Read the model definition and answer for the solid it produces. Units are mm, in the model's axes. A direction names the side the tool comes from. Coordinates: 2 decimals unless noted, no trailing zeros. Loops run counter-clockwise (first coordinate to the right, second up) from the corner with the lowest first, then second, coordinate; pieces in that order, holes last. Notation, with made-up numbers: M 41.5,77 L 88.5,77 A26 ccw 88.5,104 Z; hole C 35,54 d5. An arc over 180 degrees is marked long. One line per item, written item: value. Start each with the question number.
1. Consider probe 1 along Y at (x, z) = (-1.5, -4.5); probe 2 along Z at (x, y) = (0.5, -9); probe 3 along Z at (x, y) = (7.25, -11). Determine where each line is inside the solid, lowest interval first.
2. The part is cut by section D-D (x = -3.25). Write down the section's boundary in (y, z), then the cut area to 3 significant figures.
3. The part is cut by section C-C (y = -39.5). Write down the section's boundary in (x, z), then the cut area to 3 significant figures.
4. The part is cut by section A-A (z = 0). Write down the section's boundary in (x, y), then the cut area to 3 significant figures.
5. The part is cut by section B-B (x = 0). Write down the section's boundary in (y, z), then the cut area to 3 significant figures.
6. For faces 1 (the face through (0, 5.75, 0)), 2 (the face through (1, 2.15, 0)), determine the directions among +Z, -Z, +X, -X, +Y, -Y from which every point of the face is accessible in a straight line to the end or side of a thin tool.
7. Flat-ended cylindrical pins translate along their axes: pin 1 (1 mm diameter, centred on y = -27.5, z = -2, fed in from +X); pin 2 (1 mm diameter, centred on x = -1.5, y = -28, fed in from -Z); pin 3 (2 mm diameter, centred on x = -2.5, z = 4, fed in from +Y). Find the tip coordinate at first contact, or state that the pin passes through.
```python
from build123d import *

# Parameters (mm, degrees)
SKETCH1_R           = 8
BOSS_EXTRUDE1_DEPTH = 45
SKETCH2_R           = 2.5
BOSS_EXTRUDE2_DEPTH = 0.6
SKETCH3_R           = 0.75
BOSS_EXTRUDE3_DEPTH = 5.75
SKETCH5_R           = 1.25
BOSS_EXTRUDE4_DEPTH = 2.15


with BuildPart() as part:
    # Sketch1 → Boss-Extrude1 (new body)
    with BuildSketch(Plane(origin=(0, 0, 0), x_dir=(1, 0, 0), z_dir=(0, 1, 0))):
        with Locations(Location((0, 0, 0), (0, 0, 270))):
            Circle(SKETCH1_R)
    extrude(amount=-BOSS_EXTRUDE1_DEPTH)

    # Sketch2 → Boss-Extrude2 (add)
    with BuildSketch(Plane(origin=(0, 0, 0), x_dir=(1, 0, 0), z_dir=(0, 1, 0))):
        with Locations(Location((0, 0, 0), (0, 0, 270))):
            Circle(SKETCH2_R)
    extrude(amount=BOSS_EXTRUDE2_DEPTH)

    # Sketch3 → Boss-Extrude3 (add)
    with BuildSketch(Plane(origin=(0, 0, 0), x_dir=(1, 0, 0), z_dir=(0, 1, 0))):
        with Locations(Location((0, 0, 0), (0, 0, 270))):
            Circle(SKETCH3_R)
    extrude(amount=BOSS_EXTRUDE3_DEPTH)

    # Sketch5 → Boss-Extrude4 (add)
    with BuildSketch(Plane(origin=(0, 0, 0), x_dir=(1, 0, 0), z_dir=(0, 1, 0))):
        with Locations(Location((0, 0, 0), (0, 0, 90))):
            Circle(SKETCH5_R)
    extrude(amount=BOSS_EXTRUDE4_DEPTH)


solid = part.part
```
Answer block:
1. probe 1: y = -45 to 0
1. probe 2: z = -7.98 to 7.98
1. probe 3: z = -3.38 to 3.38
2. outline: M -45,-7.31 L 0,-7.31 L 0,7.31 L -45,7.31 Z
2. area: 658 mm2
3. outline: C 0,0 d16
3. area: 201 mm2
4. outline: M -8,-45 L 8,-45 L 8,0 L 2.5,0 L 2.5,0.6 L 1.25,0.6 L 1.25,2.15 L 0.75,2.15 L 0.75,5.75 L -0.75,5.75 L -0.75,2.15 L -1.25,2.15 L -1.25,0.6 L -2.5,0.6 L -2.5,0 L -8,0 Z
4. area: 732 mm2
5. outline: M -45,-8 L 0,-8 L 0,-2.5 L 0.6,-2.5 L 0.6,-1.25 L 2.15,-1.25 L 2.15,-0.75 L 5.75,-0.75 L 5.75,0.75 L 2.15,0.75 L 2.15,1.25 L 0.6,1.25 L 0.6,2.5 L 0,2.5 L 0,8 L -45,8 Z
5. area: 732 mm2
6. face 1: +Z, -Z, +X, -X, +Y
6. face 2: +Y
7. pin 1: stops at x = 7.86
7. pin 2: stops at z = -7.94
7. pin 3: stops at y = 0
